Check sheet for the modelled part. Datum: model origin and axes. Units: mm. A direction names the side the tool comes from. Give positions to 0.01 mm unless a question says otherwise; leave off trailing zeros. Loops run counter-clockwise (first coordinate to the right, second up) from the corner with the lowest first, then second, coordinate; pieces in that order, holes last.
```python
from build123d import *

# Parameters (mm, degrees)
BOSS_EXTRUDE1_DEPTH = 70
SKETCH2_R           = 19
CUT_EXTRUDE1_DEPTH  = 108.956316041
FILLET1_R           = 5


with BuildPart() as part:
    # Sketch1 → Boss-Extrude1 (new body)
    with BuildSketch(Plane(origin=(0, 0, 0), x_dir=(1, 0, 0), z_dir=(0, 1, 0))):
        Polygon((-37.290686498, 31.356060606), (-35.290686498, 31.356060606), (-35.290686498, -68.643939394), (4.709313502, -68.643939394), (4.709313502, -70.643939394), (-37.290686498, -70.643939394), align=None)
    extrude(amount=BOSS_EXTRUDE1_DEPTH)

    # Sketch2 → Cut-Extrude1 (cut, through all)
    with BuildSketch(Plane.ZY.offset(37.290686498)):
        with Locations((4.183939394, 35)):
            Circle(SKETCH2_R)
    extrude(amount=-CUT_EXTRUDE1_DEPTH, mode=Mode.SUBTRACT)

    # Fillet1
    fillet1_edges = [part.edges().sort_by_distance(p)[0] for p in [
        (-35.290686498, 35, 68.643939394),
        (-37.290686498, 35, 70.643939394),
    ]]
    fillet(fillet1_edges, radius=FILLET1_R)


solid = part.part
```
(1) Section check C-C on y = 12. Record the boundary of the cut face in (x, z).
(2) Section check B-B on z = 19. Record the boundary of the cut face in (x, y).
(3) Release check for a two-part mould opening along Y. For faces 3 (the face through (-36.3, 16.45, 0.07)), 4 (the face through (-36, 0, 23)), 5 (the face through (-36, 70, 23)), 6 (the face through (-13, 35, 68.644)) record: pulls with the +Y half, pulls with the -Y half, needs draft (parallel to the pull), parting line crosses it, or undercut.
(4) Material ranges on line 1 (X direction, y = 7, z = 41.5); line 2 (Z direction, x = -20, y = 34); line 3 (X direction, y = 59.5, z = 64.5), recorded low to high.
(5) Section check A-A on y = 35. Record the boundary of the cut face in (x, z).
(6) Section check D-D on z = 3.5. Record the boundary of the cut face in (x, y), plus the area to 3 significant figures.
(7) Gauge pin test, flat ends, axial feed: pin 1 Ø10.5 at (x, y) = (-9, 44.5) entering from -Z; pin 2 Ø2 at (y, z) = (20.5, 58.5) entering from +X. Record the tip position at first contact, or that the pin passes through.
(8) Access from +Z, -Z, +X, -X, +Y, -Y to the whole of each face (thin tool, end or side, straight path). Record for faces 1 (the face through (-14, 35, 70.644)), 2 (the face through (-35.291, 35, 26)).
Computed values:
1. outline: (-37.29, -31.36) - (-35.29, -31.36) - (-35.29, 63.64) arc R5 cw to (-30.29, 68.64) - (4.71, 68.64) - (4.71, 70.64) - (-32.29, 70.64) arc R5 ccw to (-37.29, 65.64) - close
2. outline: (-37.29, 0) - (-35.29, 0) - (-35.29, 23.11) - (-37.29, 23.11) - close; (-37.29, 46.89) - (-35.29, 46.89) - (-35.29, 70) - (-37.29, 70) - close
3. face 3: undercut
3. face 4: pulls with the -Y half
3. face 5: pulls with the +Y half
3. face 6: needs draft
4. line 1: x = -37.29 to -35.29
4. line 2: z = 68.64 to 70.64
4. line 3: x = -37.29 to -35.22
5. outline: (-37.29, -31.36) - (-35.29, -31.36) - (-35.29, -14.82) - (-37.29, -14.82) - close; (-37.29, 23.18) - (-35.29, 23.18) - (-35.29, 63.64) arc R5 cw to (-30.29, 68.64) - (4.71, 68.64) - (4.71, 70.64) - (-32.29, 70.64) arc R5 ccw to (-37.29, 65.64) - close
6. outline: (-37.29, 0) - (-35.29, 0) - (-35.29, 16.01) - (-37.29, 16.01) - close; (-37.29, 53.99) - (-35.29, 53.99) - (-35.29, 70) - (-37.29, 70) - close
6. area: 64.0 mm2
7. pin 1: stops at z = 68.64
7. pin 2: stops at x = -35.29
8. face 1: +Z, +X, -X, +Y, -Y
8. face 2: -Z, +X, +Y, -Y
